Source: three-view drawing plus pictorial views. Frame: mm from the lowest corner of the part. Give positions to 0.01 mm unless a question says otherwise; leave off trailing zeros. Order: outer loops, then holes, each group sorted by start corner. A loop starts at its lowest first (then second) coordinate and runs counter-clockwise, first axis right, second up.
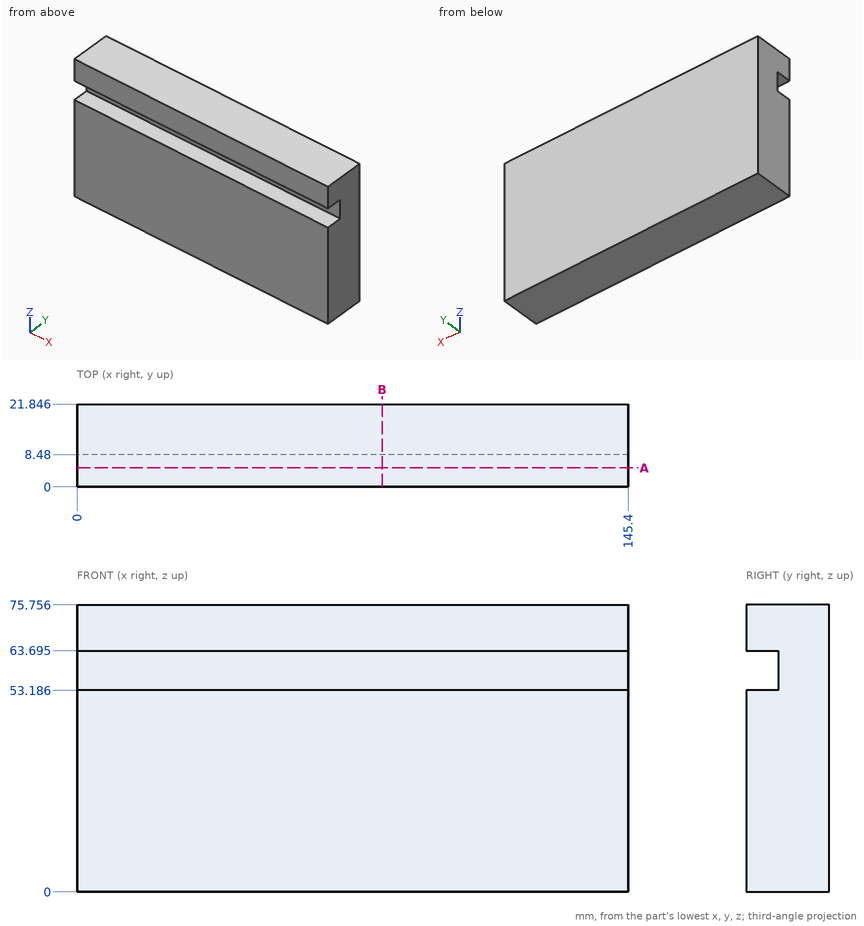
1) Section query B-B on x = 80.5. Output: boundary loops of the cut face in (y, z) (1 decimal), and give its area (3 significant figures).
Checks:
outline: (0, 0) - (21.8, 0) - (21.8, 75.8) - (0, 75.8) - (0, 63.7) - (8.5, 63.7) - (8.5, 53.2) - (0, 53.2) - close
area: 1,570 mm2
2) Ray query, L1, parallel to Z at x = 10, y = 7.5 (1 decimal); L2, parallel to Y at x = 42, z = 56. Return the intervals inside material, ascending.
Checks:
L1: z = 0 to 53.2, 63.7 to 75.8
L2: y = 8.48 to 21.85
3) Section query A-A on y = 5. Output: boundary loops of the cut face in (x, z) (1 decimal).
Checks:
outline: (0, 0) - (145.4, 0) - (145.4, 53.2) - (0, 53.2) - close; (0, 63.7) - (145.4, 63.7) - (145.4, 75.8) - (0, 75.8) - close
